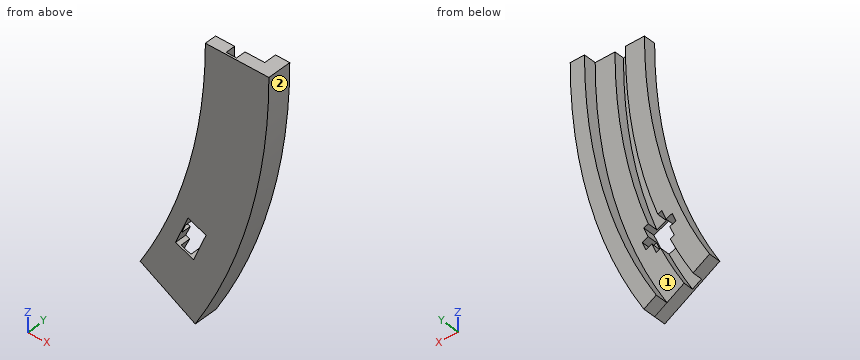
from build123d import *

# Parameters (mm, degrees)
AUFSATZ_LINEAR_AUSTRAGEN1_DEPTH = 3.6
SCHNITT_LINEAR_AUSTRAGEN1_DEPTH = 3
SCHNITT_LINEAR_AUSTRAGEN2_DEPTH = 190.652735282
SCHNITT_LINEAR_AUSTRAGEN3_DEPTH = 3
AUFSATZ_LINEAR_AUSTRAGEN2_DEPTH = 3.8


with BuildPart() as part:
    # Skizze1 → Aufsatz-Linear austragen1 (new body)
    with BuildSketch(Plane(origin=(0, 0, 0), x_dir=(1, 0, 0), z_dir=(0, 1, 0))):
        with BuildLine():
            Line((146.877908482, 84.8), (129.903810568, 75))
            ThreePointArc((129.903810568, 75), (144.888873943, 38.822856765), (150, 0))
            Line((150, 0), (169.6, 0))
            ThreePointArc((169.6, 0), (163.821020139, 43.895710049), (146.877908482, 84.8))
        make_face()
    extrude(amount=AUFSATZ_LINEAR_AUSTRAGEN1_DEPTH)

    # Skizze2 → Schnitt-Linear austragen1 (cut)
    with BuildSketch(Plane(origin=(0, 3.6, 0), x_dir=(1, 0, 0), z_dir=(0, 1, 0))):
        with BuildLine():
            Line((135.01336045, 77.95), (137.784641742, 79.55))
            ThreePointArc((137.784641742, 79.55), (153.678798963, 41.178110076), (159.1, 0))
            Line((159.1, 0), (155.9, 0))
            ThreePointArc((155.9, 0), (150.587836318, 40.349889131), (135.01336045, 77.95))
        make_face()
    extrude(amount=-SCHNITT_LINEAR_AUSTRAGEN1_DEPTH, mode=Mode.SUBTRACT)

    # Skizze3 → Schnitt-Linear austragen2 (cut, through all)
    with BuildSketch(Plane(origin=(0, 3.6, 0), x_dir=(1, 0, 0), z_dir=(0, 1, 0))):
        Polygon((140.825970611, 63.743987963), (146.369247806, 66.040088557), (150.19608213, 56.801293232), (144.652804935, 54.505192638), align=None)
    extrude(amount=-SCHNITT_LINEAR_AUSTRAGEN2_DEPTH, mode=Mode.SUBTRACT)

    # Skizze4 → Schnitt-Linear austragen3 (cut)
    with BuildSketch(Plane(origin=(0, 3.6, 0), x_dir=(1, 0, 0), z_dir=(0, 1, 0))):
        Polygon((140.317603559, 59.745042734), (149.556398885, 63.571877058), (150.704449182, 60.800238461), (141.465653857, 56.973404137), align=None)
    extrude(amount=-SCHNITT_LINEAR_AUSTRAGEN3_DEPTH, mode=Mode.SUBTRACT)

    # Skizze5 → Aufsatz-Linear austragen2 (add)
    with BuildSketch(Plane(origin=(0, 3.6, 0), x_dir=(1, 0, 0), z_dir=(0, 1, 0))):
        with BuildLine():
            Line((143.067396705, 82.6), (146.877908482, 84.8))
            ThreePointArc((146.877908482, 84.8), (163.821020139, 43.895710049), (169.6, 0))
            Line((169.6, 0), (165.2, 0))
            ThreePointArc((165.2, 0), (159.570946503, 42.756906251), (143.067396705, 82.6))
        make_face()
    extrude(amount=AUFSATZ_LINEAR_AUSTRAGEN2_DEPTH)


solid = part.part
Model file for the job. Use its own axes, mm. Face numbers are marked on the shaded views. A direction names the side the tool comes from. Give positions to 0.01 mm unless a question says otherwise; leave off trailing zeros. Order: outer loops, then holes, each group sorted by start corner. A loop starts at its lowest first (then second) coordinate and runs counter-clockwise, first axis right, second up. Notation, with made-up numbers: M -19.5,81 L -4.5,81 A37 ccw -4.5,119 Z; hole C -23.75,54 d10. An arc over 180 degrees is marked long. Put each result on its own line as item: value. Start each with the question number.
(1) Drill centre lines: L1, parallel to Y at x = 149, z = -68.5; L2, parallel to X at y = 1.5, z = -44.5; L3, parallel to X at y = 3, z = -22.5. Where is each one in solid material? Low to high. Write a range as [from, to].
(2) Band-saw the part on A-A on y = 2. Give the cut face in (x, z).
(3) Tool access for the marked faces 1 and 2: list every direction of +Z, -Z, +X, -X, +Y, -Y with a clear straight run to the whole face (end or side of a thin tool).
(4) Band-saw the part on D-D on x = 160.5. Give the cut face in (y, z), then the cut area to 3 significant figures.
(5) Band-saw the part on B-B on z = -41.5. Give the cut face in (x, y), then the cut area to 3 significant figures.
(6) Pin check, flat tips, straight feed: pin 1 Ø1.5 at (x, y) = (143, 1) entering from -Z; pin 2 Ø0.9 at (x, z) = (149.5, -62) entering from +Y; pin 3 Ø10.5 at (x, z) = (153, -20.5) entering from +Y. Stop position of each tip, or through.
Results below:
1. L1: y = [0, 3.6]
1. L2: x = [143.25, 149.41], [152.75, 163.66]
1. L3: x = [148.3, 154.27], [157.5, 168.1]
2. outline: M 129.9,-75 L 135.01,-77.95 A155.9 ccw 142.05,-64.25 L 140.83,-63.74 L 142.17,-60.51 L 140.32,-59.75 L 141.47,-56.97 L 143.31,-57.74 L 144.65,-54.51 L 145.87,-55.01 A155.9 ccw 155.9,0 L 150,0 A150 cw Z; M 137.78,-79.55 L 146.88,-84.8 A169.6 ccw 169.6,0 L 159.1,0 A159.1 cw 148.83,-56.24 L 150.2,-56.8 L 148.86,-60.03 L 150.7,-60.8 L 149.56,-63.57 L 147.71,-62.81 L 146.37,-66.04 L 145,-65.47 A159.1 cw Z
3. face 1: +Z, -X, +Y
3. face 2: -Z, +X, +Y, -Y
4. outline: M 0,-54.81 L 7.4,-54.81 L 7.4,-39.13 L 3.6,-39.13 L 3.6,0 L 0,0 Z
4. area: 257 mm2
5. outline: M 144.14,0 L 164.44,0 L 164.44,7.4 L 159.9,7.4 L 159.9,3.6 L 153.59,3.6 L 153.59,0.6 L 150.27,0.6 L 150.27,3.6 L 144.14,3.6 Z
5. area: 80.4 mm2
6. pin 1: stops at z = -82.99
6. pin 2: stops at y = 0.6
6. pin 3: stops at y = 3.6
